```python
from build123d import *

# Parameters (mm, degrees)
EXTRUDE_1_DEPTH     = 4.95
SKETCH_2_R          = 10.11
CUT_EXTRUDE_1_DEPTH = 3
CUT_EXTRUDE_2_DEPTH = 2.5
SKETCH_4_R          = 7.5
CUT_EXTRUDE_3_DEPTH = 0.6
CUT_EXTRUDE_4_REACH = 23.036
SKETCH_5_R          = 3
SKETCH_8_W          = 3.5
SKETCH_8_H          = 0.6
SKETCH_9_R          = 0.75
EXTRUDE_2_DEPTH     = 1.5
SKETCH_10_W         = 0.6
SKETCH_10_H         = 1.115
CUT_EXTRUDE_5_DEPTH = 3.5
SKETCH_16_W         = 0.6
SKETCH_16_H         = 1.27
EXTRUDE_3_DEPTH     = 3.5


with BuildPart() as part:
    # Sketch 1 → Extrude 1 (new body)
    with BuildSketch(Plane(origin=(0, 0, 0), x_dir=(1, 0, 0), z_dir=(0, 1, 0))):
        with BuildLine():
            Line((11.710705572, 3), (16.325, 3))
            ThreePointArc((16.325, 3), (17.032106781, 2.707106781), (17.325, 2))
            Line((17.325, 2), (17.325, -2))
            ThreePointArc((17.325, -2), (17.032106781, -2.707106781), (16.325, -3))
            Line((16.325, -3), (11.710705572, -3))
            ThreePointArc((11.710705572, -3), (11.128997881, -3.186602089), (10.76438593, -3.676767677))
            ThreePointArc((10.76438593, -3.676767677), (-11.375, 0), (10.76438593, 3.676767677))
            ThreePointArc((10.76438593, 3.676767677), (11.128997881, 3.186602089), (11.710705572, 3))
        make_face()
    extrude(amount=EXTRUDE_1_DEPTH)

    # Sketch 2 → Cut-Extrude 1 (cut)
    with BuildSketch(Plane(origin=(0, 4.95, 0), x_dir=(-1, 0, 0), z_dir=(0, 1, 0))):
        with Locations(Location((0, 0, 0), (0, 0, 90))):
            Circle(SKETCH_2_R)
    extrude(amount=-CUT_EXTRUDE_1_DEPTH, mode=Mode.SUBTRACT)

    # Sketch 3 → Cut-Extrude 2 (cut)
    with BuildSketch(Plane(origin=(0, 4.95, 0), x_dir=(-1, 0, 0), z_dir=(0, 1, 0))):
        with BuildLine():
            Line((8.755516832, -5.055), (9.851038968, -5.6875))
            ThreePointArc((9.851038968, -5.6875), (11.375, 0), (9.851038968, 5.6875))
            Line((9.851038968, 5.6875), (8.755516832, 5.055))
            ThreePointArc((8.755516832, 5.055), (10.11, 0), (8.755516832, -5.055))
        make_face()
    extrude(amount=-CUT_EXTRUDE_2_DEPTH, mode=Mode.SUBTRACT)

    # Sketch 4 → Cut-Extrude 3 (cut)
    with BuildSketch(Plane(origin=(0, 1.95, 0), x_dir=(-1, 0, 0), z_dir=(0, 1, 0))):
        with Locations(Location((0, 0, 0), (0, 0, 90))):
            Circle(SKETCH_4_R)
    extrude(amount=-CUT_EXTRUDE_3_DEPTH, mode=Mode.SUBTRACT)

    # Sketch 5 → Cut-Extrude 4 (cut, up to next)
    with BuildSketch(Plane(origin=(0, 1.35, 0), x_dir=(-1, 0, 0), z_dir=(0, 1, 0)), mode=Mode.PRIVATE) as cut_extrude_4_sk1:
        with Locations(Location((0, 0, 0), (0, 0, 90))):
            Circle(SKETCH_5_R)
    cut_extrude_4_tool1 = extrude(cut_extrude_4_sk1.sketch, amount=-CUT_EXTRUDE_4_REACH, mode=Mode.PRIVATE) & part.part
    add(cut_extrude_4_tool1.solids().sort_by_distance((0, 1.35, 0))[0], mode=Mode.SUBTRACT)

    # Sweep 2: sweep along a path in Sketch 7
    with BuildLine(Plane.XY) as sweep_2_path:
        Line((-6.482147214, -5), (-6.482147214, 1.15))
        ThreePointArc((-6.482147214, 1.15), (-6.335700604, 1.503553391), (-5.982147214, 1.65))
        Line((-5.982147214, 1.65), (4.458438225, 1.65))
    # Sketch 8 → Sweep 2 (sweep)
    with BuildSketch(Plane(origin=(4.458438225, 0, 0), x_dir=(0, 0, -1), z_dir=(1, 0, 0))):
        with Locations((0, 1.65)):
            Rectangle(SKETCH_8_W, SKETCH_8_H)
    sweep(path=sweep_2_path.line)

    # Sketch 9 → Extrude 2 (add)
    with BuildSketch(Plane.XZ):
        with Locations(Location((0, 9.575, 0), (0, 0, 270))):
            Circle(SKETCH_9_R)
        with Locations(Location((8.292193241, -4.7875, 0), (0, 0, 270))):
            Circle(SKETCH_9_R)
        with Locations(Location((-8.292193241, -4.7875, 0), (0, 0, 270))):
            Circle(SKETCH_9_R)
    extrude(amount=EXTRUDE_2_DEPTH)

    # Sketch 10 → Cut-Extrude 5 (cut)
    with BuildSketch(Plane.XZ.offset(5)):
        with Locations((-6.482147214, 1.1925)):
            Rectangle(SKETCH_10_W, SKETCH_10_H)
        with Locations((-6.482147214, -1.1925)):
            Rectangle(SKETCH_10_W, SKETCH_10_H)
    extrude(amount=-CUT_EXTRUDE_5_DEPTH, mode=Mode.SUBTRACT)

    # Sweep 3: sweep along a path in Sketch 12
    with BuildLine(Plane.XY) as sweep_3_path:
        Line((14.017852786, 0), (14.017852786, 4.75))
        ThreePointArc((14.017852786, 4.75), (13.871406177, 5.103553391), (13.517852786, 5.25))
        Line((13.517852786, 5.25), (7.770329112, 5.25))
        ThreePointArc((7.770329112, 5.25), (7.348318318, 5.220169505), (6.934700052, 5.13127126))
        Line((6.934700052, 5.13127126), (-2.128848466, 2.502652205))
        ThreePointArc((-2.128848466, 2.502652205), (-2.998479817, 2.384116164), (-3.865200914, 2.522333456))
        Line((-3.865200914, 2.522333456), (-5.047739274, 2.89455308))
    # Sketch 14 → Sweep 3 (sweep)
    with BuildSketch(Plane.XZ):
        Polygon((14.317852786, -1.76229338), (14.317852786, 1.73770662), (14.017852786, 1.73770662), (13.717852786, 1.73770662), (13.717852786, -1.76229338), (14.017852786, -1.76229338), align=None)
    sweep(path=sweep_3_path.line)

    # Sweep 4: sweep along a path in Sketch 15
    with BuildLine(Plane.XY) as sweep_4_path:
        Line((14.017852786, 0), (14.017852786, -1.5))
    # Sketch 14_3 → Sweep 4 (sweep)
    with BuildSketch(Plane.XZ):
        Polygon((14.317852786, -1.76229338), (14.317852786, 1.73770662), (14.017852786, 1.73770662), (13.717852786, 1.73770662), (13.717852786, -1.76229338), (14.017852786, -1.76229338), align=None)
    sweep(path=sweep_4_path.line)

    # Sketch 16 → Extrude 3 (add)
    with BuildSketch(Plane.XZ.offset(1.5)):
        with Locations((14.017852786, -0.01229338)):
            Rectangle(SKETCH_16_W, SKETCH_16_H)
    extrude(amount=EXTRUDE_3_DEPTH)


solid = part.part
```
The model under review builds one solid part; all positions refer to its coordinate system, in mm. A direction names the side the tool comes from. Give positions to 0.01 mm unless a question says otherwise; leave off trailing zeros. Loops run counter-clockwise (first coordinate to the right, second up) from the corner with the lowest first, then second, coordinate; pieces in that order, holes last. Notation, with made-up numbers: (-13.75, 75.25) - (2.25, 75.25) arc R20 cw to (2.25, 79.25) - close; hole circle Ø8 at (39, -26.75). An arc over 180 degrees is marked (long way). Answer as a JSON object with one key per item and string values.
Q1. Add section C-C on x = 5.75. State the section outline as (y, z) points.
Worked out:
{"outline": "(0, -9.81) - (4.95, -9.81) - (4.95, -8.32) - (1.95, -8.32) - (1.95, -4.82) - (1.35, -4.82) - (1.35, 4.82) - (1.95, 4.82) - (1.95, 8.32) - (4.95, 8.32) - (4.95, 9.81) - (0, 9.81) - close; (4.48, -1.76) - (5.1, -1.76) - (5.1, 1.74) - (4.48, 1.74) - close"}
Q2. Add section B-B on x = 0. State the section outline as (y, z) points (3 decimals), plus the area to 3 significant figures.
Worked out:
{"outline": "(-1.5, 8.825) - (0, 8.825) - (0, 3) - (1.35, 3) - (1.35, 7.5) - (1.95, 7.5) - (1.95, 10.11) - (4.95, 10.11) - (4.95, 11.375) - (0, 11.375) - (0, 10.325) - (-1.5, 10.325) - close; (0, -11.375) - (4.95, -11.375) - (4.95, -10.11) - (1.95, -10.11) - (1.95, -7.5) - (1.35, -7.5) - (1.35, -3) - (0, -3) - close; (1.35, -1.75) - (1.95, -1.75) - (1.95, 1.75) - (1.35, 1.75) - close; (2.808, -1.762) - (3.432, -1.762) - (3.432, 1.738) - (2.808, 1.738) - close", "area": "41.4 mm^2"}
Q3. Mouldability with a two-part tool opening along Y and no side actions: class faces 1 (the flat face through (17.325, 2, 0)), 2 (the flat face through (11, 5.55, 0)), 3 (the cylindrical face through (-3.418, 2.115, -0.037)) as +Y half, -Y half, draft (parallel to the pull), parting line (faces both ways), or undercut.
Worked out:
{"face 1": "draft", "face 2": "+Y half", "face 3": "undercut"}
Q4. To check wall thickness, follow line 1 along Z through (x, y) = (0, 1.15) (3 decimals); line 2 along X through (y, z) = (1.6, 0) (3 decimals); line 3 along X through (y, z) = (1.75, 0) (3 decimals). State the ranges of each line that lie inside material, in increasing order.
Worked out:
{"line 1": "z = -11.375 to -3, 3 to 11.375", "line 2": "x = -11.375 to -7.5, -6.644 to 4.458, 7.5 to 17.325", "line 3": "x = -11.375 to -7.5, -6.511 to 4.458, 7.5 to 17.325"}
Q5. Add section A-A on y = -3.5. State the section outline as (x, z) points (3 decimals).
Worked out:
{"outline": "(-6.782, -0.635) - (-6.182, -0.635) - (-6.182, 0.635) - (-6.782, 0.635) - close; (13.718, -0.647) - (14.318, -0.647) - (14.318, 0.623) - (13.718, 0.623) - close"}
Q6. Add section D-D on y = 1. State the section outline as (x, z) points (3 decimals).
Worked out:
{"outline": "(10.764, -3.677) arc R1 cw to (11.711, -3) - (16.325, -3) arc R1 ccw to (17.325, -2) - (17.325, 2) arc R1 ccw to (16.325, 3) - (11.711, 3) arc R1 cw to (10.764, 3.677) arc R11.375 ccw (long way) to start; hole circle Ø6 at (0, 0)"}
Q7. For faces 4 (the flat face through (14.318, -2, 0)), 5 (the flat face through (14, 2, 3)), 6 (the flat face through (-10.3, 2.45, 0.1)), 7 (the flat face through (10, 4.95, -3)), 8 (the cylindrical face through (0.9, 0.68, 2.86)), list the 3-axis set-ups (+Z, -Z, +X, -X, +Y, -Y) from which the entire face can be reached by the end or side of a thin tool; tool diameter is ignored.
Worked out:
{"face 4": "+Z, -Z, +X, -Y", "face 5": "+Z, +X, +Y, -Y", "face 6": "-X, +Y", "face 7": "+X, +Y", "face 8": "-Y"}
Q8. Insertion check: pin 1 (0.7 mm diameter, centred on x = 1, y = 1.5, fed in from +Z); pin 2 (0.7 mm diameter, centred on x = 9.5, z = -0.5, fed in from -Y); pin 3 (3 mm diameter, centred on y = -3, z = 0, fed in from +X). Each pin has a flat end and moves straight along its axis. Give the tip position at first contact, or say it passes through.
Worked out:
{"pin 1": "stops at z = 11.36", "pin 2": "stops at y = 0", "pin 3": "stops at x = 14.32"}
